Part model, mm, in its own coordinate system. Give positions to 0.01 mm unless a question says otherwise; leave off trailing zeros. Order: outer loops, then holes, each group sorted by start corner. A loop starts at its lowest first (then second) coordinate and runs counter-clockwise, first axis right, second up. Notation, with made-up numbers: (-3.75, -20.5) - (53.25, -20.5) arc R16 cw to (53.25, 7.5) - close; hole circle Ø2 at (74, -28). An arc over 180 degrees is marked (long way). Use one line per item in the form item = value. Start each with the question number.
1. Band-saw the part on B-B, the plane z = 0.2. List the corners of the cut face in (x, y) (3 decimals), plus the area to 3 significant figures.
2. Band-saw the part on C-C, the plane y = 6.5. List the corners of the cut face in (x, z).
3. Drill centre lines: line 1 (Y direction, x = -7.5, z = -0.75) (3 decimals); line 2 (X direction, y = -9, z = -0.4); line 3 (X direction, y = 16, z = 0.5). Where is each one in solid material? Low to high.
4. Band-saw the part on A-A, the plane x = 2. List the corners of the cut face in (y, z) (3 decimals).
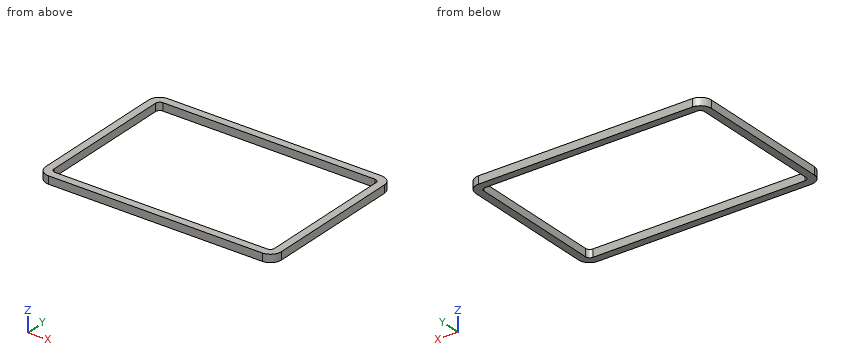
Autodesk Inventor part; units mm, degrees
ref_plane "YZ Plane" through (0, 0, 0) normal (1, 0, 0) x (0, 1, 0)
ref_plane "XZ Plane" through (0, 0, 0) normal (0, 1, 0) x (-1, 0, 0)
ref_plane "XY Plane" through (0, 0, 0) normal (0, 0, 1) x (1, 0, 0)
sketch "Sketch1" plane through (0, 0, 0) normal (0, 0, 1) x (1, 0, 0)
  line L0 (25.4, -16.637) -> (-25.4, -16.637)
  line L1 (-25.4, -16.637) -> (-25.4, 16.637)
  line L2 (-25.4, 16.637) -> (25.4, 16.637)
  line L3 (25.4, 16.637) -> (25.4, -16.637)
  line L4 (25.4, -16.637) -> (-25.4, 16.637) construction
  line L5 (-25.4, -16.637) -> (25.4, 16.637) construction
  line L6 (27.178, 18.415) -> (-27.178, 18.415)
  line L7 (-27.178, 18.415) -> (-27.178, -18.415)
  line L8 (-27.178, -18.415) -> (27.178, -18.415)
  line L9 (27.178, -18.415) -> (27.178, 18.415)
  point P0 (0, 0)
  dimension "d0" = 50.8
  dimension "d1" = 33.274
  dimension "d2" = 1.778
extrude "Extrusion1" add sketch "Sketch1" along normal mid plane 1.778
fillet "Fillet1" radius 0.9652 4 edges at (25.4, 16.637, 0) (25.4, -16.637, 0) (-25.4, -16.637, 0) (-25.4, 16.637, 0)
fillet "Fillet1" radius 2.54 4 edges at (27.178, -18.415, 0) (27.178, 18.415, 0) (-27.178, 18.415, 0) (-27.178, -18.415, 0)
properties part number "O-Ring Dash 034 Square"
From the geometry:
q1.outline = (-27.178, -15.875) arc R2.54 ccw to (-24.638, -18.415) - (24.638, -18.415) arc R2.54 ccw to (27.178, -15.875) - (27.178, 15.875) arc R2.54 ccw to (24.638, 18.415) - (-24.638, 18.415) arc R2.54 ccw to (-27.178, 15.875) - close; hole (-25.4, -15.672) arc R0.965 ccw to (-24.435, -16.637) - (24.435, -16.637) arc R0.965 ccw to (25.4, -15.672) - (25.4, 15.672) arc R0.965 ccw to (24.435, 16.637) - (-24.435, 16.637) arc R0.965 ccw to (-25.4, 15.672) - close
q1.area = 307 mm²
q2.outline = (-27.18, -0.89) - (-25.4, -0.89) - (-25.4, 0.89) - (-27.18, 0.89) - close; (25.4, -0.89) - (27.18, -0.89) - (27.18, 0.89) - (25.4, 0.89) - close
q3.line_1 = -18.415 to -16.637, 16.637 to 18.415
q3.line_2 = -27.18 to -25.4, 25.4 to 27.18
q3.line_3 = -27.17 to -25.34, 25.34 to 27.17
q4.outline = (-18.415, -0.889) - (-16.637, -0.889) - (-16.637, 0.889) - (-18.415, 0.889) - close; (16.637, -0.889) - (18.415, -0.889) - (18.415, 0.889) - (16.637, 0.889) - close
